Geometry: see drawing. Coordinates: mm, zero at the bounding-box minimum. Coordinates: 2 decimals unless noted, no trailing zeros. Order: outer loops, then holes, each group sorted by start corner. A loop starts at its lowest first (then second) coordinate and runs counter-clockwise, first axis right, second up. Notation, with made-up numbers: M 75,19.25 L 123,19.25 A12 cw 123,36.25 Z; hole C 15.5,-35 d3. An arc over 180 degrees is marked long. Answer in a Markdown table with one row per item.
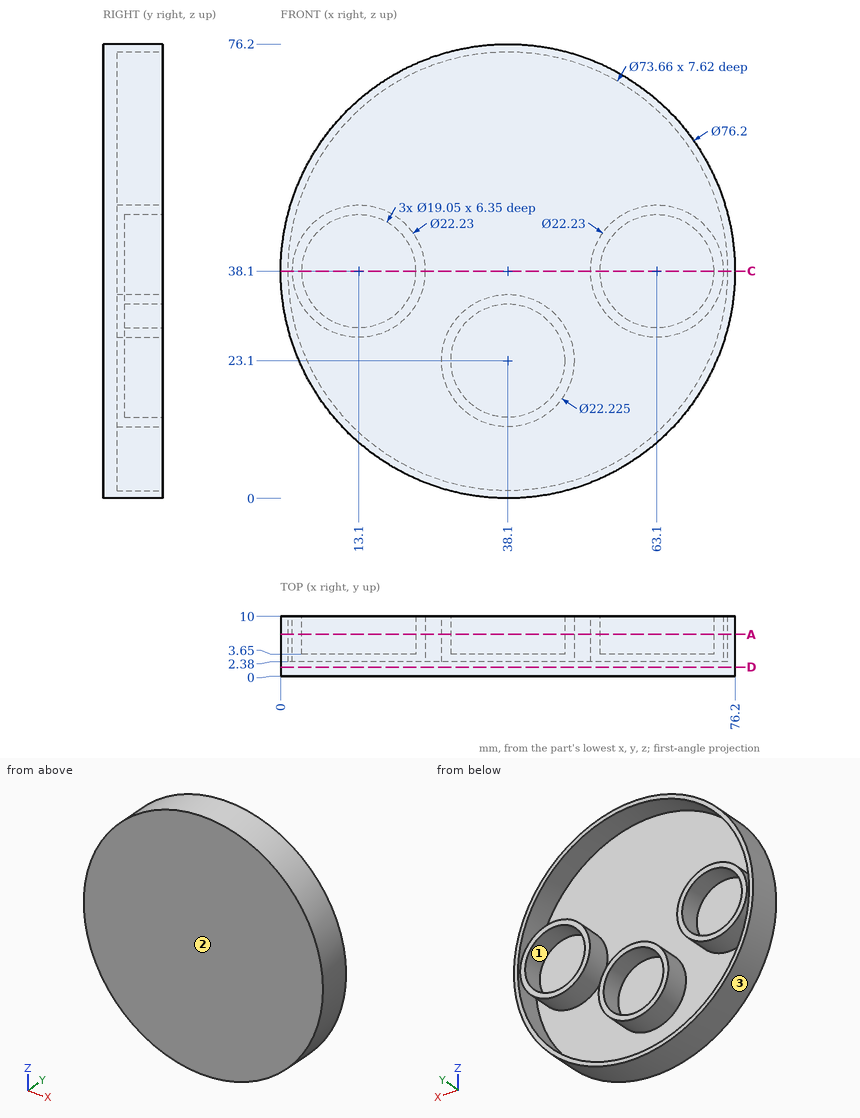
1) Mould query, pull axis X, two halves, no side actions, for the marked faces 1, 2 and 3. Classes: +X half, -X half, draft (parallel to the pull), parting line (faces both ways), or undercut.
Resolved:
| item | result |
|---|---|
| face 1 | undercut |
| face 2 | draft |
| face 3 | parting line |
2) Cut plane D-D, the plane y = 1.5. Output: boundary loops of the cut face in (x, z).
Resolved:
| item | result |
|---|---|
| outline | C 38.1,38.1 d76.2 |
3) Contact query for flat-ended pins moving along their axis: pin 1 (3 mm diameter, centred on y = 5, z = 40, fed in from -X); pin 2 (4 mm diameter, centred on x = 36.5, y = 1.5, fed in from +Z); pin 3 (5 mm diameter, centred on x = 21, y = 6, fed in from -Z). Output: stop coordinate, or through.
Resolved:
| item | result |
|---|---|
| pin 1 | stops at x = 0 |
| pin 2 | stops at z = 76.2 |
| pin 3 | stops at z = 2.91 |
4) Cut plane A-A, the plane y = 7. State how many separate pieces and enclosed holes the cut face has, and give its area (3 significant figures).
Resolved:
| item | result |
|---|---|
| separate pieces | 4 |
| enclosed holes | 4 |
| area | 608 mm2 |
5) Material intervals for probe 1 along X at (y, z) = (5, 38.1) (3 decimals); probe 2 along Z at (x, y) = (38.1, 8.25) (1 decimal); probe 3 along Z at (x, y) = (13, 4.25), sorted ascending.
Resolved:
| item | result |
|---|---|
| probe 1 | x = 0 to 1.27, 1.985 to 3.575, 22.625 to 24.215, 51.985 to 53.575, 72.625 to 74.215, 74.93 to 76.2 |
| probe 2 | z = 0 to 1.3, 12 to 13.6, 32.6 to 34.2, 74.9 to 76.2 |
| probe 3 | z = 9.44 to 11.15, 26.99 to 28.58, 47.62 to 49.21, 65.05 to 66.76 |
6) Cut plane C-C, the plane z = 38.1. Output: boundary loops of the cut face in (x, y) (3 decimals), and give its area (3 significant figures).
Resolved:
| item | result |
|---|---|
| outline | M 0,0 L 76.2,0 L 76.2,10 L 74.93,10 L 74.93,2.38 L 74.215,2.38 L 74.215,10 L 72.625,10 L 72.625,3.65 L 53.575,3.65 L 53.575,10 L 51.985,10 L 51.985,2.38 L 24.215,2.38 L 24.215,10 L 22.625,10 L 22.625,3.65 L 3.575,3.65 L 3.575,10 L 1.985,10 L 1.985,2.38 L 1.27,2.38 L 1.27,10 L 0,10 Z |
| area | 298 mm2 |
